from build123d import *

# Parameters (mm, degrees)
BOSS_EXTRU_1_START = 0.2
ESQUISSE1_R        = 1.75
BOSS_EXTRU_1_DEPTH = 3


with BuildPart() as part:
    # Esquisse1 → Boss.-Extru.1 (new body)
    with BuildSketch(Plane.XY.offset(BOSS_EXTRU_1_START)):
        with BuildLine():
            Line((0.981089506, 13.370599952), (4.55, -1.925))
            Line((4.55, -1.925), (4.55, -7.925))
            Line((4.55, -7.925), (13.55, -7.925))
            Line((13.55, -7.925), (13.55, -5.925))
            Line((13.55, -5.925), (9.357429757, -5.925))
            ThreePointArc((9.357429757, -5.925), (8.735829332, -5.708334482), (8.383587662, -5.152225822))
            Line((8.383587662, -5.152225822), (4.956202513, 9.536826262))
            ThreePointArc((4.956202513, 9.536826262), (4.968859947, 10.039957952), (5.224987097, 10.473202214))
            Line((5.224987097, 10.473202214), (8.596002843, 13.824763284))
            ThreePointArc((8.596002843, 13.824763284), (8.91971414, 14.040045447), (9.301060354, 14.115613154))
            Line((9.301060354, 14.115613154), (15, 14.115613154))
            Line((15, 14.115613154), (15, 16.615613154))
            Line((15, 16.615613154), (7.745530511, 16.588352798))
            ThreePointArc((7.745530511, 16.588352798), (6.614685245, 16.648223613), (5.49786, 16.835565296))
            Line((5.49786, 16.835565296), (4, 17.175))
            ThreePointArc((4, 17.175), (1.571663105, 16.001961319), (0.981089506, 13.370599952))
        make_face()
        with Locations((4, 14.075)):
            Circle(ESQUISSE1_R, mode=Mode.SUBTRACT)
    extrude(amount=BOSS_EXTRU_1_DEPTH)


solid = part.part
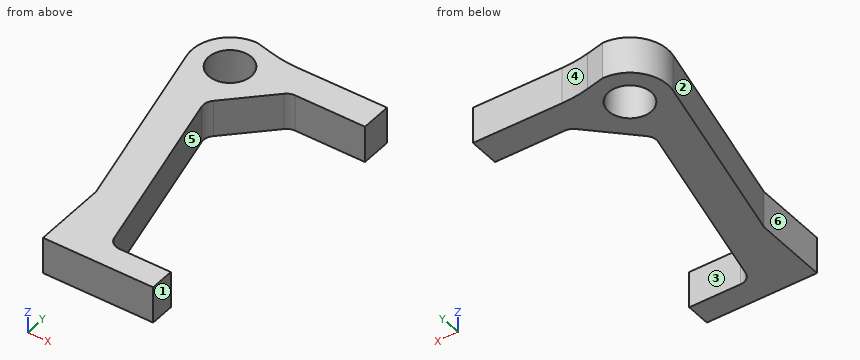
The listing builds one solid part. Answer for the finished solid, in the listing's coordinates (mm). Face numbers are marked on the shaded views. A direction names the side the tool comes from. Coordinates: 2 decimals unless noted, no trailing zeros. Order: outer loops, then holes, each group sorted by start corner. A loop starts at its lowest first (then second) coordinate and runs counter-clockwise, first axis right, second up.
Q1. Consider line 1 (Y direction, x = 9.25, z = 0.4) (3 decimals); line 2 (X direction, y = 14.75, z = 0.55); line 3 (X direction, y = 0, z = 2.7). Determine where each line is inside the solid, lowest interval first.
Q2. A cutting plane is placed at D-D, the plane y = -0.25. Write down the section's boundary in (x, z).
Q3. Which of the six approach directions +Z, -Z, +X, -X, +Y, -Y give full straight-line access (tool end or side, diameter ignored) to the marked faces 4, 5 and 6?
Q4. A cutting plane is placed at C-C, the plane x = 10. Write down the section's boundary in (y, z) (3 decimals), and give its area (3 significant figures).
Q5. For a pull along Y with two mould halves and no side action, classify the marked faces 1, 2 and 3 as pulls with the +Y half, pulls with the -Y half, needs draft (parallel to the pull), parting line crosses it, or undercut.
Q6. A cutting plane is placed at A-A, the plane x = 2.75. Write down the section's boundary in (y, z).
Q7. Given P1, Ø1, axis at x = 3, y = -3.5, coming from the -Z side; P2, Ø1, axis at y = 9, z = 2.5, coming from the -X side; P3, Ø0.9, axis at x = 12, z = 2, coming from the +Y side; P4, Ø1.6, axis at y = -7, z = 1.5, coming from the +X side, each flat-ended and moving along its own axis, determine where each tip first touches the part or whether it passes through.
Q8. A cutting plane is placed at B-B, the plane z = 2.2. Write down the section's boundary in (x, y) (3 decimals).
Answers follow:
1. line 1: y = -7.925 to -5.919, 14.114 to 16.594
1. line 2: x = 0.97 to 2.39, 5.61 to 15
1. line 3: x = 4.1 to 7.18
2. outline: (4.16, 0.2) - (7.24, 0.2) - (7.24, 3.2) - (4.16, 3.2) - close
3. face 4: +Z, -Z, +Y
3. face 5: +Z, -Z, +X
3. face 6: +Z, -Z, -X, -Y
4. outline: (-7.925, 0.2) - (-5.925, 0.2) - (-5.925, 3.2) - (-7.925, 3.2) - close; (14.116, 0.2) - (16.597, 0.2) - (16.597, 3.2) - (14.116, 3.2) - close
4. area: 13.4 mm2
5. face 1: needs draft
5. face 2: pulls with the -Y half
5. face 3: undercut
6. outline: (5.79, 0.2) - (12.85, 0.2) - (12.85, 3.2) - (5.79, 3.2) - close; (15.3, 0.2) - (16.91, 0.2) - (16.91, 3.2) - (15.3, 3.2) - close
7. P1: passes through
7. P2: stops at x = 1.88
7. P3: stops at y = 16.61
7. P4: stops at x = 13.55
8. outline: (0.981, 13.371) - (4.55, -1.925) - (4.55, -7.925) - (13.55, -7.925) - (13.55, -5.925) - (9.357, -5.925) arc R1 cw to (8.384, -5.152) - (4.956, 9.537) arc R1 cw to (5.225, 10.473) - (8.596, 13.825) arc R1 cw to (9.301, 14.116) - (15, 14.116) - (15, 16.616) - (7.746, 16.588) arc R10 cw to (5.498, 16.836) - (4, 17.175) arc R3.1 ccw to start; hole circle Ø3.5 at (4, 14.075)
